```python
from build123d import *

# Parameters (mm, degrees)
SKETCH_1_W          = 65
SKETCH_1_H          = 15
EXTRUDE_1_DEPTH     = 2
SKETCH_2_R          = 1.25
SKETCH_2_R_2        = 3.45
SKETCH_2_R_3        = 1.5
SKETCH_2_R_4        = 1
CUT_EXTRUDE_1_DEPTH = 2
SKETCH_4_R          = 1.5
EXTRUDE_2_DEPTH     = 2
SKETCH_5_R          = 7.5
SKETCH_5_R_2        = 7.1
EXTRUDE_3_DEPTH     = 8
EXTRUDE_START       = -8
SKETCH_5_5_R        = 1.25
SKETCH_5_5_R_2      = 7.1
SKETCH_5_5_R_3      = 1
SKETCH_5_5_R_4      = 1.5
EXTRUDE_4_DEPTH     = 6
CUT_EXTRUDE_START   = -5.5
SKETCH_5_6_R        = 1.25
SKETCH_5_6_R_2      = 7.1
CUT_EXTRUDE_3_DEPTH = 5.5


with BuildPart() as part:
    # 草图1 → 凸台-拉伸1 (new body)
    with BuildSketch(Plane(origin=(0, 0, 0), x_dir=(1, 0, 0), z_dir=(0, 1, 0))):
        with Locations((-7.5, 0)):
            Rectangle(SKETCH_1_W, SKETCH_1_H)
    extrude(amount=EXTRUDE_1_DEPTH)

    # 草图2 → 切除-拉伸1 (cut)
    with BuildSketch(Plane(origin=(0, 0, 0), x_dir=(1, 0, 0), z_dir=(0, 1, 0))):
        with Locations(Location((0, 0, 0), (0, 0, 270))):
            Circle(SKETCH_2_R)
        with Locations(Location((-16, 0, 0), (0, 0, 90))):
            Circle(SKETCH_2_R_2)
        with Locations(Location((-24, 0, 0), (0, 0, 90))):
            Circle(SKETCH_2_R)
        with Locations(Location((-32.5, 0, 0), (0, 0, 270))):
            Circle(SKETCH_2_R_3)
        with Locations(Location((-27, 0, 0), (0, 0, 270))):
            Circle(SKETCH_2_R_4)
        with Locations(Location((-32.5, -5.5, 0), (0, 0, 270))):
            Circle(SKETCH_2_R_4)
        with Locations(Location((-38, 0, 0), (0, 0, 270))):
            Circle(SKETCH_2_R_4)
        with Locations(Location((-32.5, 5.5, 0), (0, 0, 270))):
            Circle(SKETCH_2_R_4)
    extrude(amount=CUT_EXTRUDE_1_DEPTH, mode=Mode.SUBTRACT)

    # 草图4 → 凸台-拉伸2 (add)
    with BuildSketch(Plane.XY.offset(7.5)):
        with Locations(Location((20, 1, 0), (0, 0, 221.810314896))):
            Circle(SKETCH_4_R)
        with Locations(Location((-20, 1, 0), (0, 0, 221.810314896))):
            Circle(SKETCH_4_R)
    extrude(amount=EXTRUDE_2_DEPTH)

    # 草图5 → 凸台-拉伸3 (add)
    # profile 1 of 2: a face of its own
    with BuildSketch(Plane(origin=(0, 2, 0), x_dir=(1, 0, 0), z_dir=(0, 1, 0))):
        with Locations(Location((-32.5, 0, 0), (0, 0, 270))):
            Circle(SKETCH_5_R)
        with Locations(Location((-32.5, 0, 0), (0, 0, 270))):
            Circle(SKETCH_5_R_2, mode=Mode.SUBTRACT)
    # profile 2 of 2: a face of its own
    with BuildSketch(Plane(origin=(0, 2, 0), x_dir=(1, 0, 0), z_dir=(0, 1, 0))):
        with BuildLine():
            Line((5.149029035, -6.7), (-5.149029035, -6.7))
            ThreePointArc((-5.149029035, -6.7), (-8.45, 0), (-5.149029035, 6.7))
            Line((-5.149029035, 6.7), (5.149029035, 6.7))
            ThreePointArc((5.149029035, 6.7), (8.45, 0), (5.149029035, -6.7))
        make_face()
        with BuildLine():
            Line((4.905354218, -6), (-4.905354218, -6))
            ThreePointArc((-4.905354218, -6), (-7.75, 0), (-4.905354218, 6))
            Line((-4.905354218, 6), (4.905354218, 6))
            ThreePointArc((4.905354218, 6), (7.75, 0), (4.905354218, -6))
        make_face(mode=Mode.SUBTRACT)
    extrude(amount=-EXTRUDE_3_DEPTH)

    # 草图5<5> → 凸台-拉伸4 (add)
    # profile 1 of 2: a face of its own
    with BuildSketch(Plane(origin=(0, 2, 0), x_dir=(1, 0, 0), z_dir=(0, 1, 0)).offset(EXTRUDE_START)):
        with BuildLine():
            Line((4.905354218, -6), (-4.905354218, -6))
            ThreePointArc((-4.905354218, -6), (-7.75, 0), (-4.905354218, 6))
            Line((-4.905354218, 6), (4.905354218, 6))
            ThreePointArc((4.905354218, 6), (7.75, 0), (4.905354218, -6))
        make_face()
        with Locations(Location((0, 0, 0), (0, 0, 270))):
            Circle(SKETCH_5_5_R, mode=Mode.SUBTRACT)
    # profile 2 of 2: a face of its own
    with BuildSketch(Plane(origin=(0, 2, 0), x_dir=(1, 0, 0), z_dir=(0, 1, 0)).offset(EXTRUDE_START)):
        with Locations((-32.5, 0)):
            Circle(SKETCH_5_5_R_2)
        with Locations(Location((-32.5, 5.5, 0), (0, 0, 270))):
            Circle(SKETCH_5_5_R_3, mode=Mode.SUBTRACT)
        with Locations(Location((-38, 0, 0), (0, 0, 270))):
            Circle(SKETCH_5_5_R_3, mode=Mode.SUBTRACT)
        with Locations(Location((-32.5, 0, 0), (0, 0, 270))):
            Circle(SKETCH_5_5_R_4, mode=Mode.SUBTRACT)
        with Locations(Location((-27, 0, 0), (0, 0, 270))):
            Circle(SKETCH_5_5_R_3, mode=Mode.SUBTRACT)
        with Locations(Location((-32.5, -5.5, 0), (0, 0, 270))):
            Circle(SKETCH_5_5_R_3, mode=Mode.SUBTRACT)
    extrude(amount=EXTRUDE_4_DEPTH)

    # 草图5<6> → 切除-拉伸3 (cut)
    # profile 1 of 2: a face of its own
    with BuildSketch(Plane(origin=(0, 2, 0), x_dir=(1, 0, 0), z_dir=(0, 1, 0)).offset(CUT_EXTRUDE_START)):
        with BuildLine():
            Line((4.905354218, -6), (-4.905354218, -6))
            ThreePointArc((-4.905354218, -6), (-7.75, 0), (-4.905354218, 6))
            Line((-4.905354218, 6), (4.905354218, 6))
            ThreePointArc((4.905354218, 6), (7.75, 0), (4.905354218, -6))
        make_face()
        with Locations(Location((0, 0, 0), (0, 0, 270))):
            Circle(SKETCH_5_6_R, mode=Mode.SUBTRACT)
    # profile 2 of 2: a face of its own
    with BuildSketch(Plane(origin=(0, 2, 0), x_dir=(1, 0, 0), z_dir=(0, 1, 0)).offset(CUT_EXTRUDE_START)):
        with Locations(Location((-32.5, 0, 0), (0, 0, 270))):
            Circle(SKETCH_5_6_R_2)
    extrude(amount=CUT_EXTRUDE_3_DEPTH, mode=Mode.SUBTRACT)


solid = part.part
```
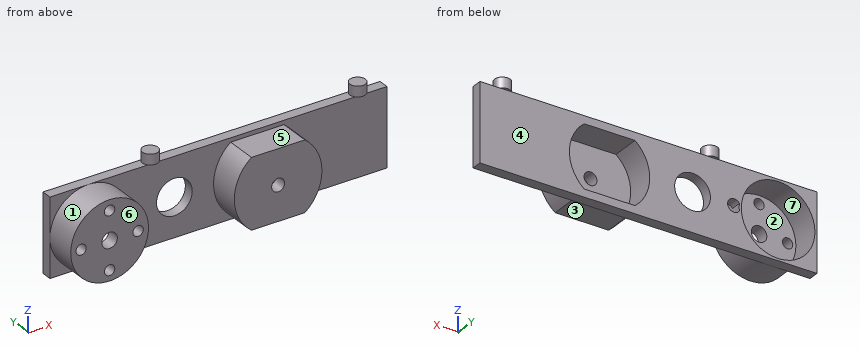
The model under review builds one solid part; all positions refer to its coordinate system, in mm. Face numbers are marked on the shaded views. A direction names the side the tool comes from. Round coordinates to 2 decimals unless told otherwise and drop trailing zeros. Order: outer loops, then holes, each group sorted by start corner. A loop starts at its lowest first (then second) coordinate and runs counter-clockwise, first axis right, second up. Notation, with made-up numbers: M 66.25,50.25 L 92.25,50.25 A35 cw 92.25,88.25 Z; hole C 75.5,51.5 d1. An arc over 180 degrees is marked long. Use a Markdown table: item, result.
1) Consider section C-C (x = -27). Write out the cut boundary in (y, z), then the cut area to 3 significant figures.
Report:
| item | result |
|---|---|
| outline | M -6,-5.1 L 0,-5.1 L 0,-7.5 L 2,-7.5 L 2,-4.49 L -3.5,-4.49 L -3.5,-1 L -6,-1 Z; M -6,1 L -3.5,1 L -3.5,4.49 L 2,4.49 L 2,7.5 L 0,7.5 L 0,5.1 L -6,5.1 Z |
| area | 36.8 mm^2 |
2) Consider section A-A (y = -4.5). Write out the cut boundary in (x, z), then the cut area to 3 significant figures.
Report:
| item | result |
|---|---|
| outline | C -32.5,0 d15; M -5.15,-6.7 L 5.15,-6.7 A8.45 ccw 5.15,6.7 L -5.15,6.7 A8.45 ccw Z; hole C -38,0 d2; hole C -32.5,0 d3; hole C -32.5,-5.5 d2; hole C -32.5,5.5 d2; hole C -27,0 d2; hole C 0,0 d2.5 |
| area | 352 mm^2 |
3) Consider section B-B (x = -6). Write out the cut boundary in (y, z), then the cut area to 3 significant figures.
Report:
| item | result |
|---|---|
| outline | M -6,-5.95 L 0,-5.95 L 0,-7.5 L 2,-7.5 L 2,-4.91 L -3.5,-4.91 L -3.5,4.91 L 2,4.91 L 2,7.5 L 0,7.5 L 0,5.95 L -6,5.95 Z |
| area | 47.4 mm^2 |
4) Wall thickness on line 1 along Z through (x, y) = (-32.5, -4.7); line 2 along Z through (x, y) = (1.5, 1.25); line 3 along X through (y, z) = (-2.5, 0.75): over which ranges is each line inside the solid? List them lowest first. Write a range as [from, to].
Report:
| item | result |
|---|---|
| line 1 | [-7.5, -6.5], [-4.5, -1.5], [1.5, 4.5], [6.5, 7.5] |
| line 2 | [-7.5, -6], [6, 7.5] |
| line 3 | [-39.96, -39.56], [-25.44, -25.04], [-8.42, -7.71], [7.71, 8.42] |
5) Insertion check: pin 1 (2 mm diameter, centred on y = -4, z = 4.5, fed in from +X); pin 2 (5 mm diameter, centred on x = 14, y = -4, fed in from +Z); pin 3 (4 mm diameter, centred on x = 0, z = 0, fed in from +Y); pin 4 (10 mm diameter, centred on x = 9.5, z = 6.5, fed in from +Y). Each pin has a flat end and moves straight along its axis. Give the tip position at first contact, or say it passes through.
Report:
| item | result |
|---|---|
| pin 1 | x = 7.69 |
| pin 2 | through |
| pin 3 | y = -3.5 |
| pin 4 | y = 2 |
6) Draft analysis for pull direction X (two halves, no side actions). For the marked faces 6 and 7, state which applies: released by +X, released by -X, zero draft, split by the parting line, or undercut.
Report:
| item | result |
|---|---|
| face 6 | zero draft |
| face 7 | undercut |
7) Tool access review of the marked faces 1, 2, 3, 4 and 5: name each direction out of +Z, -Z, +X, -X, +Y, -Y from which nothing blocks a thin tool from reaching the whole face with its end or side.
Report:
| item | result |
|---|---|
| face 1 | -Y |
| face 2 | +Y |
| face 3 | -Z, +X, -Y |
| face 4 | -Z, +X, -X, +Y |
| face 5 | +Z, +X, -Y |
8) Consider section D-D (x = -20). Write out the cut boundary in (y, z), then the cut area to 3 significant figures.
Report:
| item | result |
|---|---|
| outline | M -0.5,7.5 L 0,7.5 L 0,-7.5 L 2,-7.5 L 2,7.5 L 2.5,7.5 L 2.5,9.5 L -0.5,9.5 Z |
| area | 36.0 mm^2 |
